Source: CAD feature listing. Evaluate the final solid. Frame: model axes, mm. Face numbers are marked on the shaded views. A direction names the side the tool comes from. Give positions to 0.01 mm unless a question says otherwise; leave off trailing zeros. Write each loop counter-clockwise with the first axis right and the second up, starting at its lowest first coordinate (ties: lowest second). Pieces come first, ordered by that corner, then holes. Notation, with made-up numbers: (1.5, 22) - (58.5, 22) arc R20 ccw to (58.5, 55) - close; hole circle Ø10 at (46, 56.25). An arc over 180 degrees is marked (long way). Answer as a JSON object with one key per item and string values. Group by question number.
from build123d import *

# Parameters (mm, degrees)
SKETCH1_R           = 1.27
BOSS_EXTRUDE1_DEPTH = 9.525
SKETCH2_R           = 3.175
BOSS_EXTRUDE2_DEPTH = 2.54
FILLET1_R           = 2.032
CUT_EXTRUDE1_DEPTH  = 2.032


with BuildPart() as part:
    # Sketch1 → Boss-Extrude1 (new body, symmetric)
    with BuildSketch(Plane(origin=(0, 0, 0), x_dir=(1, 0, 0), z_dir=(0, 1, 0))):
        Circle(SKETCH1_R)
    extrude(amount=BOSS_EXTRUDE1_DEPTH, both=True)

    # Sketch2 → Boss-Extrude2 (add)
    with BuildSketch(Plane(origin=(0, 9.525, 0), x_dir=(1, 0, 0), z_dir=(0, 1, 0))):
        Circle(SKETCH2_R)
    extrude(amount=BOSS_EXTRUDE2_DEPTH)

    # Fillet1
    fillet1_edges = [part.edges().sort_by_distance(p)[0] for p in [
        (-3.175, 12.065, 0),
    ]]
    fillet(fillet1_edges, radius=FILLET1_R)

    # Sketch3 → Cut-Extrude1 (cut)
    with BuildSketch(Plane(origin=(0, 12.065, 0), x_dir=(1, 0, 0), z_dir=(0, 1, 0))):
        with BuildLine():
            Line((-0.635, 1.143), (-0.635, 2.685389765))
            Line((-0.635, 2.685389765), (0.635, 2.685389765))
            Line((0.635, 2.685389765), (0.635, 1.143))
            ThreePointArc((0.635, 1.143), (0.783789755, 0.783789755), (1.143, 0.635))
            Line((1.143, 0.635), (2.371299226, 0.635))
            Line((2.371299226, 0.635), (2.371299226, -0.635))
            Line((2.371299226, -0.635), (1.143, -0.635))
            ThreePointArc((1.143, -0.635), (0.783789755, -0.783789755), (0.635, -1.143))
            Line((0.635, -1.143), (0.635, -2.685389765))
            Line((0.635, -2.685389765), (-0.635, -2.685389765))
            Line((-0.635, -2.685389765), (-0.635, -1.143))
            ThreePointArc((-0.635, -1.143), (-0.783789755, -0.783789755), (-1.143, -0.635))
            Line((-1.143, -0.635), (-2.371299226, -0.635))
            Line((-2.371299226, -0.635), (-2.371299226, 0.635))
            Line((-2.371299226, 0.635), (-1.143, 0.635))
            ThreePointArc((-1.143, 0.635), (-0.783789755, 0.783789755), (-0.635, 1.143))
        make_face()
    extrude(amount=-CUT_EXTRUDE1_DEPTH, mode=Mode.SUBTRACT)


solid = part.part
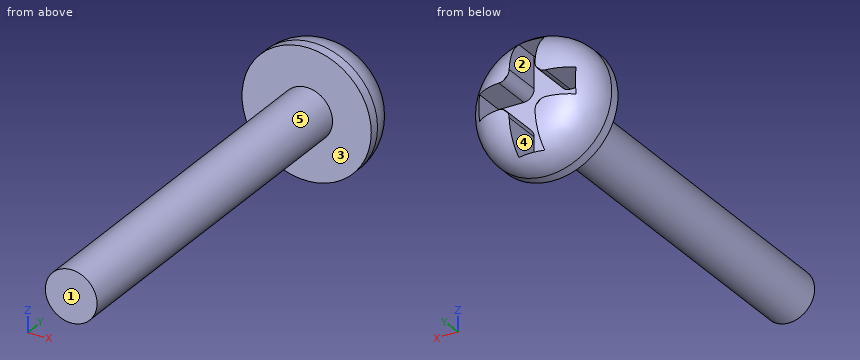
Q1. Section A-A on y = -8. Return the cut outline in (x, z).
Q2. First-contact query: pin 1 Ø1.4 at (x, z) = (0, 1) entering from +Y (3 decimals); pin 2 Ø1.4 at (x, y) = (0.5, 11) entering from +Z; pin 3 Ø1.5 at (x, y) = (0.5, 1.5) entering from +Z; pin 4 Ø0.8 at (y, z) = (10.5, 1.5) entering from -X. Flat tips, straight axial feed; report the tip coordinate or a pass-through.
Q3. Draft query along X for the marked faces 3, 4 and 5. Return one class per face: released by +X, released by -X, zero draft, split by the parting line, or undercut.
Q4. Ray query, probe 1 along Y at (x, z) = (-1, -0.5) (3 decimals); probe 2 along Y at (x, z) = (2.25, -0.5) (3 decimals); probe 3 along X at (y, z) = (-4, 1). Return the intervals inside material, ascending. Write a range as [from, to].
Q5. Reachability of the marked faces 1 and 2 from +Z, -Z, +X, -X, +Y, -Y: full face, straight path, thin tool, end or side. Return the list, or none.
Taken from the geometry:
{
 "1": {"outline": "circle Ø2.54 at (0, 0)"},
 "2": {"pin 1": "stops at y = 12.065", "pin 2": "stops at z = 3.14", "pin 3": "stops at z = 1.27", "pin 4": "stops at x = -2.94"},
 "3": {"face 3": "zero draft", "face 4": "undercut", "face 5": "split by the parting line"},
 "4": {"probe 1": "y = [-9.525, 10.033]", "probe 2": "y = [9.525, 10.033]", "probe 3": "x = [-0.78, 0.78]"},
 "5": {"face 1": "+Z, -Z, +X, -X, -Y", "face 2": "+Y"}
}
